from build123d import *

# Parameters (mm, degrees)
F0_W     = 40
F0_H     = 31
F1_DEPTH = 8.7
F2_W     = 40
F2_H     = 22
F3_DEPTH = 14.54
F4_R     = 1
F5_DEPTH = 0.5


with BuildPart() as f1:
    # F0 (on Top) → F1 (new body)
    with BuildSketch(Plane.XY):
        Rectangle(F0_W, F0_H)
    extrude(amount=F1_DEPTH)

    # F2 (on face) → F3 (join)
    with BuildSketch(Plane.XY.offset(8.7)):
        with Locations((0, 4.5)):
            Rectangle(F2_W, F2_H)
    extrude(amount=F3_DEPTH)

    # F4 (on face) → F5 (cut)
    with BuildSketch(Plane.XY.offset(8.7)):
        with Locations((0, -10.1)):
            Circle(F4_R)
    extrude(amount=-F5_DEPTH, mode=Mode.SUBTRACT)


solid = f1.part
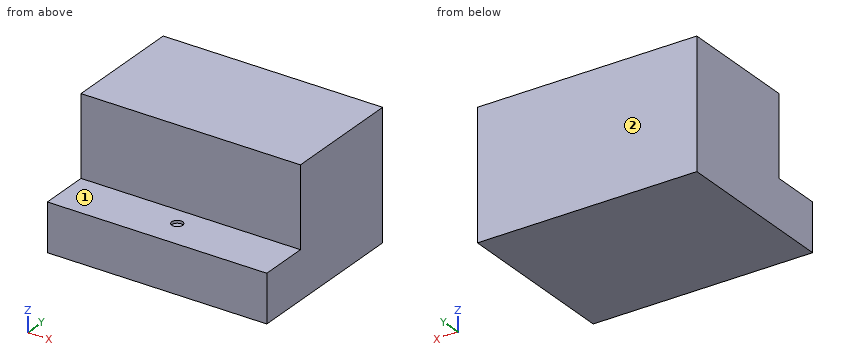
Can you work these out from the model? Positions are in its coordinate system, mm. Face numbers are marked on the shaded views. A direction names the side the tool comes from. Give positions to 0.01 mm unless a question says otherwise; leave off trailing zeros. Order: outer loops, then holes, each group sorted by start corner. A loop starts at its lowest first (then second) coordinate and runs counter-clockwise, first axis right, second up. Notation, with made-up numbers: M -4,29 L 13,29 A15 cw 13,58 Z; hole C 31,-31 d7. An arc over 180 degrees is marked long. One line per question, with ' | ' between items.
Item 1: I'm going to push flat-ended pins straight in: pin 1 Ø0.6 at (x, y) = (0, -10) entering from +Z; pin 2 Ø1.5 at (x, z) = (8, 17) entering from -Y; pin 3 Ø2.5 at (x, y) = (-5, -11) entering from +Z. Where does each tip first touch, or does it pass through?
Answer block:
pin 1: stops at z = 8.2 | pin 2: stops at y = -6.5 | pin 3: stops at z = 8.7
Item 2: Suppose I cut it at D-D, the plane x = 0. Write out the boundary of the cut face in (y, z).
Answer block:
outline: M -15.5,0 L 15.5,0 L 15.5,23.24 L -6.5,23.24 L -6.5,8.7 L -9.1,8.7 L -9.1,8.2 L -11.1,8.2 L -11.1,8.7 L -15.5,8.7 Z
Item 3: Suppose I cut it at A-A, the plane y = -10.1. Write out the boundary of the cut face in (x, z), then the cut area to 3 significant figures.
Answer block:
outline: M -20,0 L 20,0 L 20,8.7 L 1,8.7 L 1,8.2 L -1,8.2 L -1,8.7 L -20,8.7 Z | area: 347 mm2
Item 4: Suppose I cut it at C-C, the plane z = 10. Write out the boundary of the cut face in (x, y).
Answer block:
outline: M -20,-6.5 L 20,-6.5 L 20,15.5 L -20,15.5 Z
Item 5: Please list where these lines run through material, in increasing order: L1, parallel to Y at x = 0, z = 8.5; L2, parallel to Z at x = -1.5, y = -8; L3, parallel to Y at x = -7, z = 19.25.
Answer block:
L1: y = -15.5 to -11.1, -9.1 to 15.5 | L2: z = 0 to 8.7 | L3: y = -6.5 to 15.5
Item 6: Suppose I cut it at B-B, the plane x = 14. Write out the boundary of the cut face in (y, z).
Answer block:
outline: M -15.5,0 L 15.5,0 L 15.5,23.24 L -6.5,23.24 L -6.5,8.7 L -15.5,8.7 Z
Item 7: For the marked faces 1 and 2, which set-ups out of +Z, -Z, +X, -X, +Y, -Y let a thin tool reach every point of the face, with its end or its side?
Answer block:
face 1: +Z, +X, -X, -Y | face 2: +Z, -Z, +X, -X, +Y
